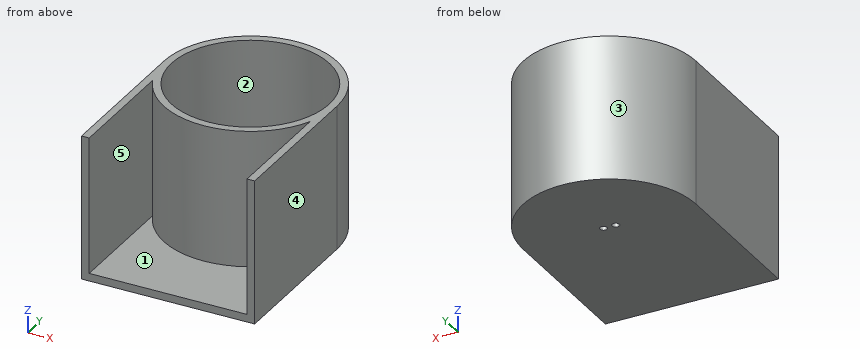
```python
from build123d import *

# Parameters (mm, degrees)
BOSS_EXTRUDE1_DEPTH            = 30
CUT_EXTRUDE1_DEPTH             = 27
SKETCH4_R                      = 0.75
CUT_EXTRUDE2_DEPTH             = 46.57411546
SKETCH5_W                      = 5
SKETCH5_H                      = 2
BOSS_EXTRUDE2_DEPTH            = 4
SHELL1_START                   = 1.6
SHELL1_DEPTH                   = 26.8
CUT_EXTRUDE3_REACH             = 49.413
CUT_EXTRUDE3_DIRECTION_2_DEPTH = 48.413078365


# Read off the part's stored shape, not the designer's step: Shell1
with BuildPart() as part:
    # Sketch2 → Boss-Extrude1 (new body)
    with BuildSketch(Plane.XY):
        with BuildLine():
            Line((-18, 0), (-18, -32))
            Line((-18, -32), (18, -32))
            Line((18, -32), (18, 0))
            ThreePointArc((18, 0), (0, 18), (-18, 0))
        make_face()
    extrude(amount=BOSS_EXTRUDE1_DEPTH)

    # Sketch3 → Cut-Extrude1 (cut)
    with BuildSketch(Plane.XY.offset(30)):
        with BuildLine():
            ThreePointArc((-16.4, 0), (0, -16.4), (16.4, 0))
            ThreePointArc((16.4, 0), (0, 16.4), (-16.4, 0))
        make_face()
    extrude(amount=-CUT_EXTRUDE1_DEPTH, mode=Mode.SUBTRACT)

    # Sketch4 → Cut-Extrude2 (cut, through all)
    with BuildSketch(Plane.XY.offset(3)):
        with Locations((-1.27, 0)):
            Circle(SKETCH4_R)
        with Locations((1.27, 0)):
            Circle(SKETCH4_R)
    extrude(amount=-CUT_EXTRUDE2_DEPTH, mode=Mode.SUBTRACT)

    # Sketch5 → Boss-Extrude2 (add)
    with BuildSketch(Plane.XY.offset(3)):
        with Locations((0, -2.475)):
            Rectangle(SKETCH5_W, SKETCH5_H)
    extrude(amount=BOSS_EXTRUDE2_DEPTH)

    # Shell1 outline → Shell1 (cut)
    with BuildSketch(Plane.XY.offset(SHELL1_START)):
        with BuildLine():
            ThreePointArc((16.4, -7.418894796), (0, -18), (-16.4, -7.418894796))
            Line((-16.4, -7.418894796), (-16.4, -32))
            Line((-16.4, -32), (16.4, -32))
            Line((16.4, -32), (16.4, -7.418894796))
        make_face()
    extrude(amount=SHELL1_DEPTH, mode=Mode.SUBTRACT)

    # Sketch6 → Cut-Extrude3 (cut, up to next)
    with BuildSketch(Plane.XY.offset(30), mode=Mode.PRIVATE) as cut_extrude3_sk1:
        with BuildLine():
            Line((-16.4, -32), (16.4, -32))
            Line((16.4, -32), (16.4, -7.418894796))
            ThreePointArc((16.4, -7.418894796), (0, -18), (-16.4, -7.418894796))
            Line((-16.4, -7.418894796), (-16.4, -32))
        make_face()
    cut_extrude3_tool1 = extrude(cut_extrude3_sk1.sketch, amount=-CUT_EXTRUDE3_REACH, mode=Mode.PRIVATE) & part.part
    add(cut_extrude3_tool1.solids().sort_by_distance((0, -23.265352, 30))[0], mode=Mode.SUBTRACT)

    # Sketch6 → Cut-Extrude3 direction 2 (cut)
    with BuildSketch(Plane.XY.offset(30)):
        with BuildLine():
            Line((-16.4, -32), (16.4, -32))
            Line((16.4, -32), (16.4, -7.418894796))
            ThreePointArc((16.4, -7.418894796), (0, -18), (-16.4, -7.418894796))
            Line((-16.4, -7.418894796), (-16.4, -32))
        make_face()
    extrude(amount=CUT_EXTRUDE3_DIRECTION_2_DEPTH, mode=Mode.SUBTRACT)


solid = part.part
```
Can you work these out from the model? Positions are in its coordinate system, mm. Face numbers are marked on the shaded views. A direction names the side the tool comes from. Coordinates: 2 decimals unless noted, no trailing zeros. Loops run counter-clockwise (first coordinate to the right, second up) from the corner with the lowest first, then second, coordinate; pieces in that order, holes last.
1) Imagine slicing it at C-C on x = -8. List the corners of the cut face in (y, z) for me.
2) Imagine slicing it at D-D on x = 1.27. List the corners of the cut face in (y, z) for me (3 decimals), plus the area to 3 significant figures.
3) Thinking about a two-plate mould opening in Y: for the marked faces 1, 2 and 3, which applies, pulls with the +Y half, pulls with the -Y half, needs draft (parallel to the pull), parting line crosses it, or undercut?
4) I need wall thicknesses on probe 1 along Y at (x, z) = (0, 3.25) (3 decimals); probe 2 along Y at (x, z) = (0, 23.25); probe 3 along Z at (x, y) = (11, -3). Which ranges of each line are inside material? Lowest first, please.
5) Imagine slicing it at B-B on z = 8. List the corners of the cut face in (x, y) for me.
6) Imagine slicing it at A-A on y = -19. List the corners of the cut face in (x, z) for me, plus the area to 3 significant figures.
7) Which directions (+Z, -Z, +X, -X, +Y, -Y) give clear straight access to the entire face, cutting with the end or side of a thin tool? Please do the marked faces 4 and 5.
8) For pin 1 (2.5 mm diameter, centred on x = -1.27, y = 0, fed in from +Z); pin 2 (2 mm diameter, centred on x = -1, z = 5.5, fed in from -Y); pin 3 (10 mm diameter, centred on x = -1.5, y = 0.5, fed in from +Z); pin 4 (1.2 mm diameter, centred on x = 1.27, y = 0, fed in from +Z), each with a flat end and sliding along its axis, tell me the tip position at first contact or that it passes through.
Completed:
1. outline: (-32, 0) - (16.12, 0) - (16.12, 30) - (14.32, 30) - (14.32, 3) - (-14.32, 3) - (-14.32, 30) - (-16.12, 30) - (-16.12, 1.6) - (-32, 1.6) - close
2. outline: (-32, 0) - (-0.75, 0) - (-0.75, 3) - (-1.475, 3) - (-1.475, 7) - (-3.475, 7) - (-3.475, 3) - (-16.351, 3) - (-16.351, 30) - (-17.955, 30) - (-17.955, 1.6) - (-32, 1.6) - close; (0.75, 0) - (17.955, 0) - (17.955, 30) - (16.351, 30) - (16.351, 3) - (0.75, 3) - close
2. area: 220 mm2
3. face 1: needs draft
3. face 2: undercut
3. face 3: pulls with the +Y half
4. probe 1: y = -18 to -16.4, -3.475 to -1.475, 16.4 to 18
4. probe 2: y = -18 to -16.4, 16.4 to 18
4. probe 3: z = 0 to 3
5. outline: (-18, -32) - (-16.4, -32) - (-16.4, -7.42) arc R18 ccw to (16.4, -7.42) - (16.4, -32) - (18, -32) - (18, 0) arc R18 ccw to (-18, 0) - close; hole circle Ø32.8 at (0, 0)
6. outline: (-18, 0) - (18, 0) - (18, 30) - (16.4, 30) - (16.4, 1.6) - (-16.4, 1.6) - (-16.4, 30) - (-18, 30) - close
6. area: 148 mm2
7. face 4: +Z, -Z, +X, +Y, -Y
7. face 5: +Z, -Y
8. pin 1: stops at z = 3
8. pin 2: stops at y = -18
8. pin 3: stops at z = 7
8. pin 4: passes through
